Input: dimensioned drawing with shaded views. Units: mm. Origin: part minimum x, y, z. Coordinates: 2 decimals unless noted, no trailing zeros. Order: outer loops, then holes, each group sorted by start corner. A loop starts at its lowest first (then second) coordinate and runs counter-clockwise, first axis right, second up. Notation, with made-up numbers: (70.25, 62) -> (75.25, 62) arc R12 cw to (75.25, 84) -> close; hole circle Ø1 at (-35.5, -13.75). An arc over 180 degrees is marked (long way). Answer as CSV lines item,"result".
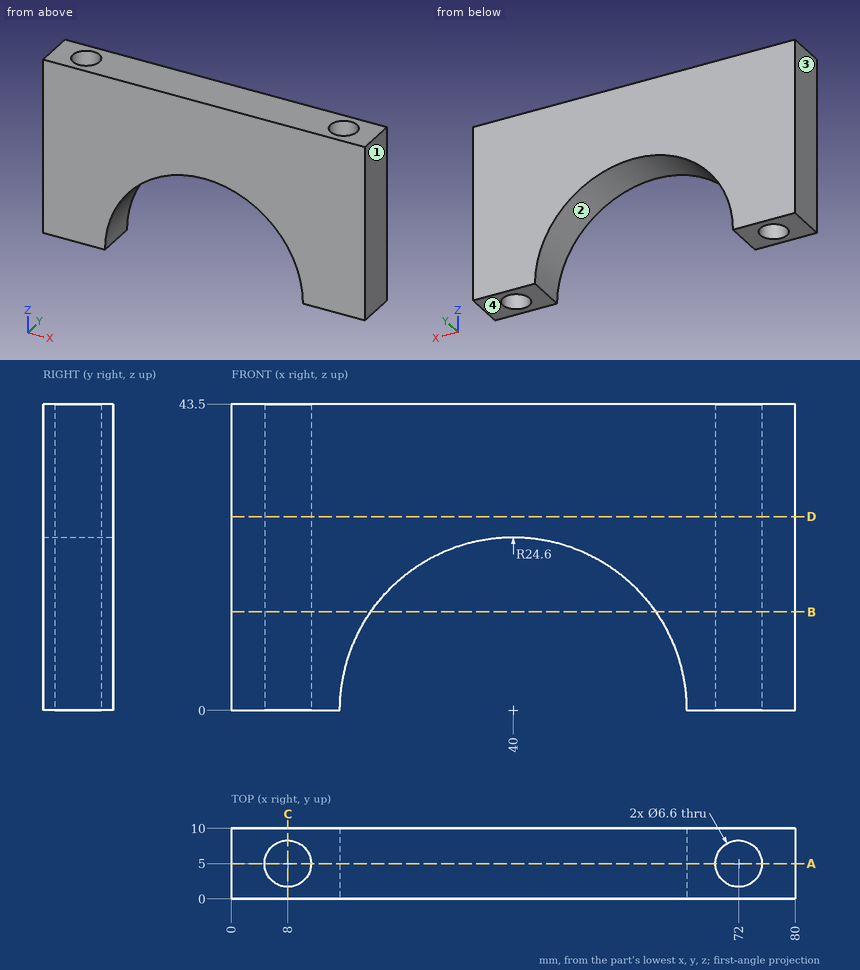
1. Mould query, pull axis X, two halves, no side actions, for the marked faces 1, 2, 3 and 4. Classes: released by +X, released by -X, zero draft, split by the parting line, or undercut.
Findings:
face 1,"released by +X"
face 2,"undercut"
face 3,"released by -X"
face 4,"zero draft"
2. Contact query for flat-ended pins moving along their axis: pin 1 (1 mm diameter, centred on x = 36, y = 8, fed in from -Z); pin 2 (1 mm diameter, centred on x = 48.5, z = 28.5, fed in from -Y). Output: stop coordinate, or through.
Findings:
pin 1,"stops at z = 24.18"
pin 2,"stops at y = 0"
3. Cut plane C-C (x = 8). Return the cut outline in (y, z), plus the area to 3 significant figures.
Findings:
outline,"(0, 0) -> (1.7, 0) -> (1.7, 43.5) -> (0, 43.5) -> close; (8.3, 0) -> (10, 0) -> (10, 43.5) -> (8.3, 43.5) -> close"
area,"148 mm2"
4. Cut plane B-B (z = 14). Return the cut outline in (x, y), plus the area to 3 significant figures.
Findings:
outline,"(0, 0) -> (19.77, 0) -> (19.77, 10) -> (0, 10) -> close; (60.23, 0) -> (80, 0) -> (80, 10) -> (60.23, 10) -> close; hole circle Ø6.6 at (8, 5); hole circle Ø6.6 at (72, 5)"
area,"327 mm2"
5. Ray query, line 1 along Y through (x, z) = (8, 20); line 2 along X through (y, z) = (7.5, 25.5); line 3 along Y through (x, z) = (11, 37.5). Return the intervals inside material, ascending.
Findings:
line 1,"y = 0 to 1.7, 8.3 to 10"
line 2,"x = 0 to 5.85, 10.15 to 69.85, 74.15 to 80"
line 3,"y = 0 to 3.63, 6.37 to 10"
6. Cut plane D-D (z = 27.5). Return the cut outline in (x, y).
Findings:
outline,"(0, 0) -> (80, 0) -> (80, 10) -> (0, 10) -> close; hole circle Ø6.6 at (8, 5); hole circle Ø6.6 at (72, 5)"
7. Cut plane A-A (y = 5). Return the cut outline in (x, z), plus the area to 3 significant figures.
Findings:
outline,"(0, 0) -> (4.7, 0) -> (4.7, 43.5) -> (0, 43.5) -> close; (11.3, 0) -> (15.4, 0) arc R24.6 cw to (64.6, 0) -> (68.7, 0) -> (68.7, 43.5) -> (11.3, 43.5) -> close; (75.3, 0) -> (80, 0) -> (80, 43.5) -> (75.3, 43.5) -> close"
area,"1,960 mm2"
